Part print with two shaded views. Sizes in mm from the minimum x, y, z corner. A direction names the side the tool comes from. Coordinates: 2 decimals unless noted, no trailing zeros. Order: outer loops, then holes, each group sorted by start corner. A loop starts at its lowest first (then second) coordinate and runs counter-clockwise, first axis right, second up. Notation, with made-up numbers: M 78,16.5 L 103,16.5 A23 cw 103,31.5 Z; hole C -4,-4 d5. An arc over 180 degrees is marked long. Answer in a Markdown table with one row per item. Add a question column.
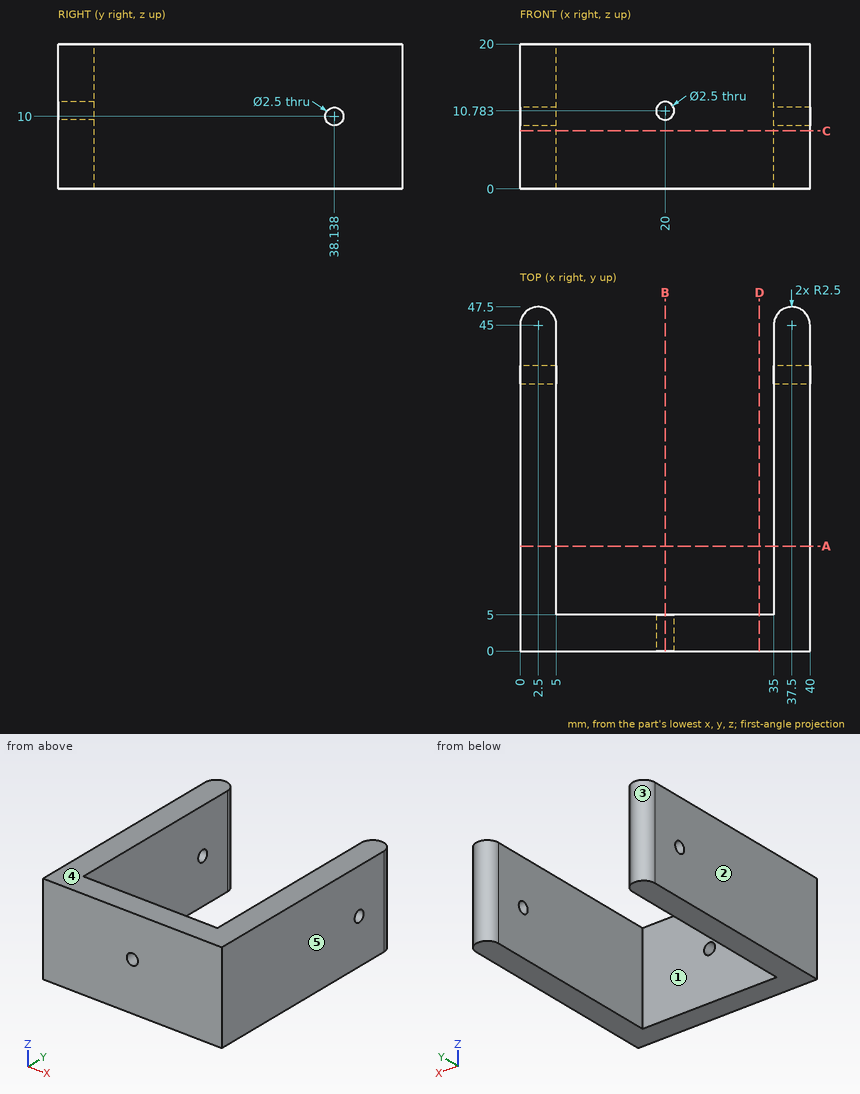
(1) Slice it at C-C (z = 8). List the corners of the cut face in (x, y).
(2) Slice it at B-B (x = 20). List the corners of the cut face in (y, z).
(3) Pull direction X, two halves, no side cores. Call the marked faces 3, 4 and 5: pulls with the +X half, pulls with the -X half, needs draft (parallel to the pull), parting line crosses it, or undercut.
(4) Slice it at A-A (y = 14.5). List the corners of the cut face in (x, z), and give its area (3 significant figures).
(5) Drop flat-ended pins along their axis: P1, Ø5, axis at x = 6.5, z = 14, coming from the +Y side; P2, Ø1.5, axis at x = 20, z = 10.78, coming from the +Y side; P3, Ø6, axis at x = 27, z = 11, coming from the +Y side. Give the stop position or say it passes through.
(6) Slice it at D-D (x = 33). List the corners of the cut face in (y, z), and give its area (3 significant figures).
(7) 3-axis set-ups, long thin cutter, end or side, ignore diameter. For the marked faces 1 and 2: which of +Z, -Z, +X, -X, +Y, -Y reach the whole face in a straight line?
(8) Wall check: line 1 (X direction, y = 32.5, z = 9.75); line 2 (Y direction, x = 18.5, z = 15.75); line 3 (Z direction, x = 19.5, y = 3.5). Give the ranges that are in metal, low to high.
Computed:
| question | item | result |
|---|---|---|
| 1 | outline | M 0,0 L 40,0 L 40,45 A2.5 ccw 35,45 L 35,5 L 5,5 L 5,45 A2.5 ccw 0,45 Z |
| 2 | outline | M 0,0 L 5,0 L 5,9.53 L 0,9.53 Z; M 0,12.03 L 5,12.03 L 5,20 L 0,20 Z |
| 3 | face 3 | undercut |
| 3 | face 4 | needs draft |
| 3 | face 5 | pulls with the +X half |
| 4 | outline | M 0,0 L 5,0 L 5,20 L 0,20 Z; M 35,0 L 40,0 L 40,20 L 35,20 Z |
| 4 | area | 200 mm^2 |
| 5 | P1 | stops at y = 47 |
| 5 | P2 | passes through |
| 5 | P3 | stops at y = 5 |
| 6 | outline | M 0,0 L 5,0 L 5,20 L 0,20 Z |
| 6 | area | 100 mm^2 |
| 7 | face 1 | +Z, -Z, +Y |
| 7 | face 2 | +Z, -Z, -X, +Y, -Y |
| 8 | line 1 | x = 0 to 5, 35 to 40 |
| 8 | line 2 | y = 0 to 5 |
| 8 | line 3 | z = 0 to 9.64, 11.93 to 20 |
